The figure shows three views and two pictorial views of one solid part (mm, origin at its lowest corner). Answer the questions. A direction names the side the tool comes from. Coordinates: 2 decimals unless noted, no trailing zeros. Order: outer loops, then holes, each group sorted by start corner. A loop starts at its lowest first (then second) coordinate and runs counter-clockwise, first axis right, second up. Notation, with made-up numbers: M 33,59 L 65,59 A23 ccw 65,76 Z; hole C 44,-28 d1. An arc over 180 degrees is marked long. Write item = value, one per line. Start each with the question number.
Q1. Straight lines are drawn through the part: line 1 along X through (y, z) = (18.5, 3.75); line 2 along Y through (x, z) = (2.5, 15.5). For each, find the intervals that lie inside material, in ascending order.
Q2. Find section D-D on x = 13.75. Give the vertices of the cut face in (y, z).
Q3. Each of these flat-tipped pins is pushed along its axis until it touches: P1, Ø1.5, axis at x = 2.5, z = 17, coming from the +Y side; P2, Ø0.6, axis at x = 19.5, z = 19, coming from the +Y side; P3, Ø1.5, axis at x = 6, y = 8.5, coming from the +Z side. Where does it stop, or does it pass through?
Q4. Find section B-B on y = 13.5. Give the vertices of the cut face in (x, z), and give its area (3 significant figures).
Q5. Find section C-C on z = 8. Give the vertices of the cut face in (x, y), and give its area (3 significant figures).
Q6. Find section A-A on x = 10. Give the vertices of the cut face in (y, z), and give its area (3 significant figures).
Q7. A tool of negligible diameter and unlimited length cuts with its end or side. For the marked faces 1, 2 and 3, from which of +Z, -Z, +X, -X, +Y, -Y can it reach the whole face along a straight path? Write none if from no direction.
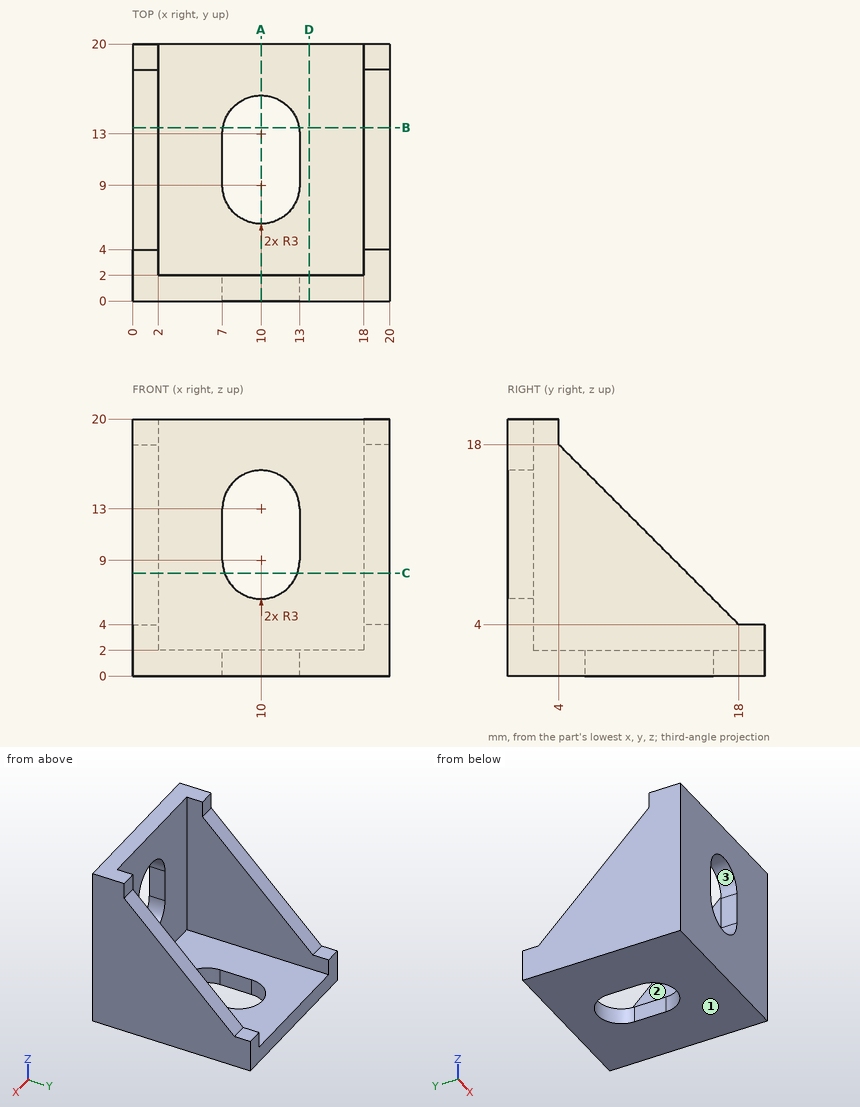
Findings below:
q1.line_1 = 0 to 2, 18 to 20
q1.line_2 = 0 to 2
q2.outline = M 0,0 L 20,0 L 20,2 L 2,2 L 2,20 L 0,20 Z
q3.P1 = 5.56
q3.P2 = 4
q3.P3 = 2
q4.outline = M 0,0 L 7.04,0 L 7.04,2 L 2,2 L 2,8.5 L 0,8.5 Z; M 12.96,0 L 20,0 L 20,8.5 L 18,8.5 L 18,2 L 12.96,2 Z
q4.area = 54.2 mm^2
q5.outline = M 0,0 L 7.17,0 L 7.17,2 L 2,2 L 2,14 L 0,14 Z; M 12.83,0 L 20,0 L 20,14 L 18,14 L 18,2 L 12.83,2 Z
q5.area = 76.7 mm^2
q6.outline = M 0,0 L 6,0 L 6,2 L 2,2 L 2,6 L 0,6 Z; M 0,16 L 2,16 L 2,20 L 0,20 Z; M 16,0 L 20,0 L 20,2 L 16,2 Z
q6.area = 36.0 mm^2
q7.face_1 = -Z, +X, -X, +Y, -Y
q7.face_2 = +Z, +Y
q7.face_3 = +Y, -Y
